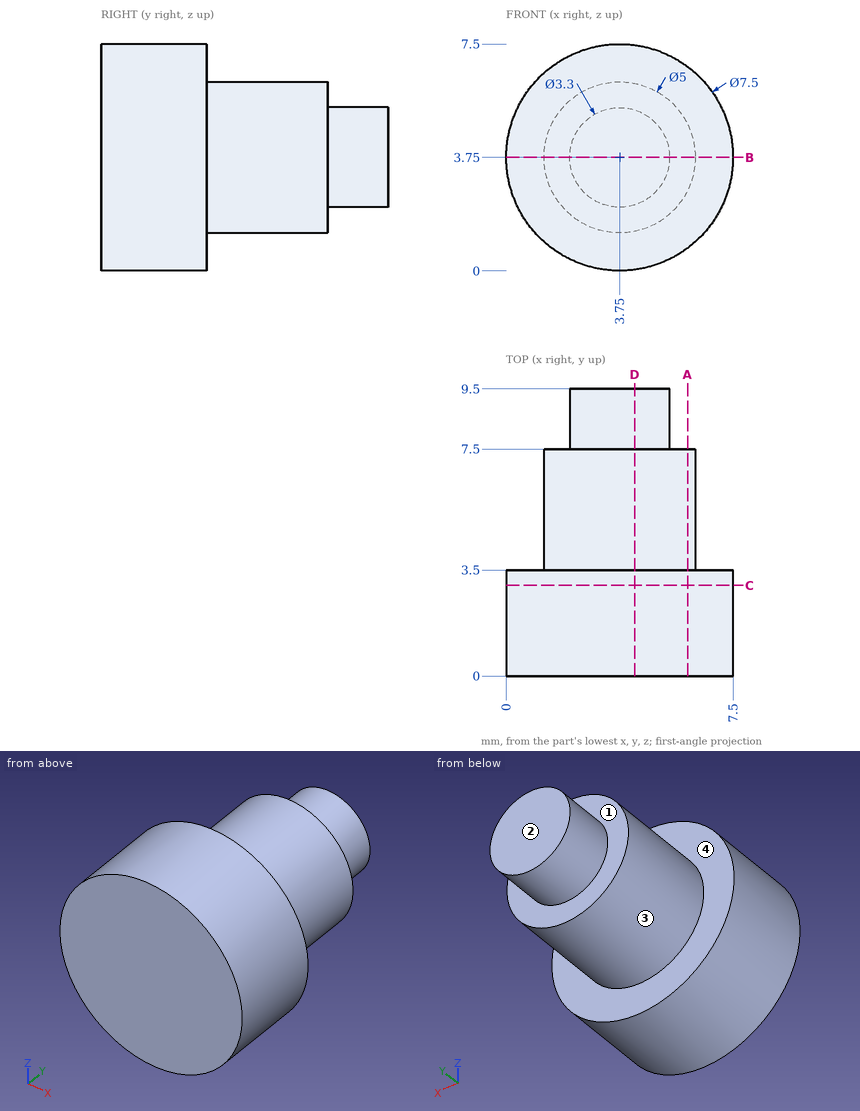
Answer from the drawing. Dimensions are ordinates in mm from the lowest x, y and z of the part. A direction names the side the tool comes from. Give positions to 0.01 mm unless a question says otherwise; leave off trailing zeros. Loops run counter-clockwise (first coordinate to the right, second up) from the corner with the lowest first, then second, coordinate; pieces in that order, holes last.
Item 1: The part is cut by section C-C (y = 3). Write down the section's boundary in (x, z), and give its area (3 significant figures).
Item 2: The part is cut by section B-B (z = 3.75). Write down the section's boundary in (x, y), and give its area (4 significant figures).
Item 3: The mould has two halves that part along X. Classify the marked faces 3 and 4: released by +X, released by -X, zero draft, split by the parting line, or undercut.
Item 4: The part is cut by section D-D (x = 4.25). Write down the section's boundary in (y, z).
Item 5: Each of these flat-tipped pins is pushed along its axis until it touches: pin 1 Ø3 at (x, y) = (3, 3.5) entering from -Z; pin 2 Ø4 at (x, y) = (4.5, 8.5) entering from +Z; pin 3 Ø2 at (x, y) = (1, 3) entering from +Z; pin 4 Ø4 at (y, z) = (5, 2) entering from -X. Where does it stop, or does it pass through?
Item 6: The part is cut by section A-A (x = 6). Write down the section's boundary in (y, z), and give its area (3 significant figures).
Item 7: For the marked faces 1 and 2, determine the directions among +Z, -Z, +X, -X, +Y, -Y from which every point of the face is accessible in a straight line to the end or side of a thin tool.
Item 8: Find the intervals of material crossed by line 1 along Y through (x, z) = (1.25, 3.25); line 2 along Y through (x, z) = (5.5, 2); line 3 along Z through (x, y) = (3.75, 4.25), in increasing order.
Taken from the geometry:
1. outline: circle Ø7.5 at (3.75, 3.75)
1. area: 44.2 mm2
2. outline: (0, 0) - (7.5, 0) - (7.5, 3.5) - (6.25, 3.5) - (6.25, 7.5) - (5.4, 7.5) - (5.4, 9.5) - (2.1, 9.5) - (2.1, 7.5) - (1.25, 7.5) - (1.25, 3.5) - (0, 3.5) - close
2. area: 52.85 mm2
3. face 3: split by the parting line
3. face 4: zero draft
4. outline: (0, 0.03) - (3.5, 0.03) - (3.5, 1.3) - (7.5, 1.3) - (7.5, 2.18) - (9.5, 2.18) - (9.5, 5.32) - (7.5, 5.32) - (7.5, 6.2) - (3.5, 6.2) - (3.5, 7.47) - (0, 7.47) - close
5. pin 1: stops at z = 0
5. pin 2: stops at z = 6.25
5. pin 3: stops at z = 7.07
5. pin 4: stops at x = 0.02
6. outline: (0, 0.75) - (3.5, 0.75) - (3.5, 2.66) - (7.5, 2.66) - (7.5, 4.84) - (3.5, 4.84) - (3.5, 6.75) - (0, 6.75) - close
6. area: 29.7 mm2
7. face 1: +Y
7. face 2: +Z, -Z, +X, -X, +Y
8. line 1: y = 0 to 3.5
8. line 2: y = 0 to 7.5
8. line 3: z = 1.25 to 6.25
